from build123d import *

# Parameters (mm, degrees)
F0_R     = 1.5
F0_R_2   = 1.3
F1_DEPTH = 38.5
F2_DEPTH = 1
F3_START = -0.5
F3_DEPTH = 0.5
F4_DEPTH = 10
F5_SIZE  = 0.2
F6_SIZE  = 0.1


with BuildPart() as f1:
    # F0 (on Top) → F1 (new body)
    with BuildSketch(Plane.XY):
        Circle(F0_R)
        Circle(F0_R_2, mode=Mode.SUBTRACT)
        Circle(F0_R_2)
    extrude(amount=F1_DEPTH)

    # F0 (on Top) → F2 (join)
    with BuildSketch(Plane.XY):
        Circle(F0_R_2)
    extrude(amount=-F2_DEPTH)

    # F0 (on Top) → F3 (join)
    with BuildSketch(Plane.XY.offset(F3_START)):
        Circle(F0_R)
        Circle(F0_R_2, mode=Mode.SUBTRACT)
    extrude(amount=-F3_DEPTH)

    # F4 (add): a face of the model
    f4_faces = [f1.faces().sort_by_distance(p)[0] for p in [
        (0, 0, -1),
    ]]
    extrude(f4_faces, amount=F4_DEPTH)

    # F5
    f5_edges = [f1.edges().sort_by_distance(p)[0] for p in [
        (-1.5, 0, 38.5),
        (-1.5, 0, -11),
    ]]
    chamfer(f5_edges, length=F5_SIZE)

    # F6
    f6_edges = [f1.edges().sort_by_distance(p)[0] for p in [
        (-1.5, 0, -0.5),
        (-1.5, 0, 0),
    ]]
    chamfer(f6_edges, length=F6_SIZE)


solid = f1.part
Verification items for the finished model (mm, model axes). A direction names the side the tool comes from. Coordinates: 2 decimals unless noted, no trailing zeros. Loops run counter-clockwise (first coordinate to the right, second up) from the corner with the lowest first, then second, coordinate; pieces in that order, holes last. Notation, with made-up numbers: (71.5, 8) -> (124.5, 8) arc R23 ccw to (124.5, 36) -> close; hole circle Ø6 at (-10.75, 59.25). An arc over 180 degrees is marked (long way). Answer as a JSON object with one key per item and string values. Group by question number.
Item 1: Sectioned sample at A-A on z = -5. Record the boundary of the cut face in (x, y).
Item 2: Depth check by flat-ended pin: pin 1 (1 mm diameter, centred on y = 1, z = 25.5, fed in from -X); pin 2 (1 mm diameter, centred on x = -1, z = 11, fed in from -Y). Enter the tip coordinate at first touch or a pass-through.
Item 3: Tool access check on faces 1 (the cylindrical face through (-1.5, 0.07, 18.93)), 2 (the cylindrical face through (-0.17, 1.29, -0.25)). Record the directions out of +Z, -Z, +X, -X, +Y, -Y that give a thin tool (end or side, any length) a straight path to the whole face; none if there is none.
Item 4: Scan lines: probe 1 along Z at (x, y) = (1.2, -0.7); probe 2 along Y at (x, z) = (1.05, 34); probe 3 along Y at (x, z) = (0.85, 28). Record each from-to range of solid material in increasing order.
Evaluation:
{
 "1": {"outline": "circle Ø3 at (0, 0)"},
 "2": {"pin 1": "stops at x = -1.41", "pin 2": "stops at y = -1.41"},
 "3": {"face 1": "+Z, -Z", "face 2": "none"},
 "4": {"probe 1": "z = -10.91 to -0.5, 0 to 38.41", "probe 2": "y = -1.07 to 1.07", "probe 3": "y = -1.24 to 1.24"}
}
